CAD build for the part. Positions are in the model's coordinates, mm. A direction names the side the tool comes from. Give positions to 0.01 mm unless a question says otherwise; leave off trailing zeros. Order: outer loops, then holes, each group sorted by start corner. A loop starts at its lowest first (then second) coordinate and runs counter-clockwise, first axis right, second up.
Item 1: Two-plate mould, pull along X, no slides. Class faces 1 (the flat face through (-1.386, 0.74, 5.223)), 2 (the flat face through (0.1, 0, 2.5)), 3 (the flat face through (-5.328, 0.74, 0.835)): released by +X, released by -X, zero draft, split by the parting line, or undercut.
Item 2: Band-saw the part on A-A on x = 0. Give the cut face in (y, z).
Item 3: Which spindle directions (+Z, -Z, +X, -X, +Y, -Y) get a long thin tool onto all of the face, cutting with end or side? Do faces 4 (the flat face through (2.44, 0.74, 4.81)), 5 (the flat face through (-1.387, 0.74, -5.211)), 6 (the flat face through (-5.34, 0.74, -0.83)), 7 (the flat face through (1.387, 0.74, 5.211)). Say none if no direction does.
Item 4: Band-saw the part on B-B on z = -1.5. Give the cut face in (x, y), plus the area to 3 significant figures.
Item 5: Flat gauge pins, fed straight in: P1, Ø3.5, axis at x = 0, z = 0, coming from the -Y side; P2, Ø2, axis at x = -4, z = 2.5, coming from the -Y side. Where does each tip first touch, or does it go through?
Item 6: Wall check: L1, parallel to X at y = 0.5, z = 0; L2, parallel to Z at x = 0.5, y = 1.1; L3, parallel to Z at x = -1, y = 0.15. Give the ranges that are in metal, low to high.
```python
from build123d import *

# Parameters (mm, degrees)
BOSS_EXTRUDE1_DEPTH = 1.5
SKETCH2_R           = 2
CUT_EXTRUDE1_DEPTH  = 9.326084366


with BuildPart() as part:
    # Sketch1 → Boss-Extrude1 (new body)
    with BuildSketch(Plane(origin=(0, 0, 0), x_dir=(1, 0, 0), z_dir=(0, 1, 0))):
        with BuildLine():
            Line((-0.133547548, 5.8), (0.133547548, 5.8))
            Line((0.133547548, 5.8), (0.408993174, 4.983244383))
            ThreePointArc((0.408993174, 4.983244383), (0.522642316, 4.972609477), (0.636019074, 4.959383))
            Line((0.636019074, 4.959383), (1.075258593, 5.701022181))
            Line((1.075258593, 5.701022181), (1.33651702, 5.645489988))
            Line((1.33651702, 5.645489988), (1.436130457, 4.789314075))
            ThreePointArc((1.436130457, 4.789314075), (1.545084972, 4.755282581), (1.653234236, 4.718772781))
            Line((1.653234236, 4.718772781), (2.237070774, 5.352882336))
            Line((2.237070774, 5.352882336), (2.481074286, 5.244244973))
            Line((2.481074286, 5.244244973), (2.400501948, 4.38606776))
            ThreePointArc((2.400501948, 4.38606776), (2.5, 4.330127019), (2.598195129, 4.271929549))
            Line((2.598195129, 4.271929549), (3.301112228, 4.770795846))
            Line((3.301112228, 4.770795846), (3.517196699, 4.613801288))
            Line((3.517196699, 4.613801288), (3.259959985, 3.791129237))
            ThreePointArc((3.259959985, 3.791129237), (3.345653032, 3.715724127), (3.429602427, 3.638382497))
            Line((3.429602427, 3.638382497), (4.220879236, 3.980202686))
            Line((4.220879236, 3.980202686), (4.399600739, 3.781712348))
            Line((4.399600739, 3.781712348), (3.976942128, 3.030500175))
            ThreePointArc((3.976942128, 3.030500175), (4.045084972, 2.938926261), (4.111119642, 2.84582067))
            Line((4.111119642, 2.84582067), (4.956173568, 3.015655569))
            Line((4.956173568, 3.015655569), (5.089721116, 2.784344431))
            Line((5.089721116, 2.784344431), (4.520112816, 2.137423713))
            ThreePointArc((4.520112816, 2.137423713), (4.567727288, 2.033683215), (4.612961202, 1.928882825))
            Line((4.612961202, 1.928882825), (5.474859333, 1.919309833))
            Line((5.474859333, 1.919309833), (5.557396256, 1.665287302))
            Line((5.557396256, 1.665287302), (4.865732884, 1.150931578))
            ThreePointArc((4.865732884, 1.150931578), (4.890738004, 1.039558454), (4.913194221, 0.927643544))
            Line((4.913194221, 0.927643544), (5.754267473, 0.739081047))
            Line((5.754267473, 0.739081047), (5.782186513, 0.473449127))
            Line((5.782186513, 0.473449127), (4.998697077, 0.114138211))
            ThreePointArc((4.998697077, 0.114138211), (5, 0), (4.998697077, -0.114138211))
            Line((4.998697077, -0.114138211), (5.782186513, -0.473449127))
            Line((5.782186513, -0.473449127), (5.754267473, -0.739081047))
            Line((5.754267473, -0.739081047), (4.913194221, -0.927643544))
            ThreePointArc((4.913194221, -0.927643544), (4.890738004, -1.039558454), (4.865732884, -1.150931578))
            Line((4.865732884, -1.150931578), (5.557396256, -1.665287302))
            Line((5.557396256, -1.665287302), (5.474859333, -1.919309833))
            Line((5.474859333, -1.919309833), (4.612961202, -1.928882825))
            ThreePointArc((4.612961202, -1.928882825), (4.567727288, -2.033683215), (4.520112816, -2.137423713))
            Line((4.520112816, -2.137423713), (5.089721116, -2.784344431))
            Line((5.089721116, -2.784344431), (4.956173568, -3.015655569))
            Line((4.956173568, -3.015655569), (4.111119642, -2.84582067))
            ThreePointArc((4.111119642, -2.84582067), (4.045084972, -2.938926261), (3.976942128, -3.030500175))
            Line((3.976942128, -3.030500175), (4.399600739, -3.781712348))
            Line((4.399600739, -3.781712348), (4.220879236, -3.980202686))
            Line((4.220879236, -3.980202686), (3.429602427, -3.638382497))
            ThreePointArc((3.429602427, -3.638382497), (3.345653032, -3.715724127), (3.259959985, -3.791129237))
            Line((3.259959985, -3.791129237), (3.517196699, -4.613801288))
            Line((3.517196699, -4.613801288), (3.301112228, -4.770795846))
            Line((3.301112228, -4.770795846), (2.598195129, -4.271929549))
            ThreePointArc((2.598195129, -4.271929549), (2.5, -4.330127019), (2.400501948, -4.38606776))
            Line((2.400501948, -4.38606776), (2.481074286, -5.244244973))
            Line((2.481074286, -5.244244973), (2.237070774, -5.352882336))
            Line((2.237070774, -5.352882336), (1.653234236, -4.718772781))
            ThreePointArc((1.653234236, -4.718772781), (1.545084972, -4.755282581), (1.436130457, -4.789314075))
            Line((1.436130457, -4.789314075), (1.33651702, -5.645489988))
            Line((1.33651702, -5.645489988), (1.075258593, -5.701022181))
            Line((1.075258593, -5.701022181), (0.636019074, -4.959383))
            ThreePointArc((0.636019074, -4.959383), (0.522642316, -4.972609477), (0.408993174, -4.983244383))
            Line((0.408993174, -4.983244383), (0.133547548, -5.8))
            Line((0.133547548, -5.8), (-0.133547548, -5.8))
            Line((-0.133547548, -5.8), (-0.408993174, -4.983244383))
            ThreePointArc((-0.408993174, -4.983244383), (-0.522642316, -4.972609477), (-0.636019074, -4.959383))
            Line((-0.636019074, -4.959383), (-1.075258593, -5.701022181))
            Line((-1.075258593, -5.701022181), (-1.33651702, -5.645489988))
            Line((-1.33651702, -5.645489988), (-1.436130457, -4.789314075))
            ThreePointArc((-1.436130457, -4.789314075), (-1.545084972, -4.755282581), (-1.653234236, -4.718772781))
            Line((-1.653234236, -4.718772781), (-2.237070774, -5.352882336))
            Line((-2.237070774, -5.352882336), (-2.481074286, -5.244244973))
            Line((-2.481074286, -5.244244973), (-2.400501948, -4.38606776))
            ThreePointArc((-2.400501948, -4.38606776), (-2.5, -4.330127019), (-2.598195129, -4.271929549))
            Line((-2.598195129, -4.271929549), (-3.301112228, -4.770795846))
            Line((-3.301112228, -4.770795846), (-3.517196699, -4.613801288))
            Line((-3.517196699, -4.613801288), (-3.259959985, -3.791129237))
            ThreePointArc((-3.259959985, -3.791129237), (-3.345653032, -3.715724127), (-3.429602427, -3.638382497))
            Line((-3.429602427, -3.638382497), (-4.220879236, -3.980202686))
            Line((-4.220879236, -3.980202686), (-4.399600739, -3.781712348))
            Line((-4.399600739, -3.781712348), (-3.976942128, -3.030500175))
            ThreePointArc((-3.976942128, -3.030500175), (-4.045084972, -2.938926261), (-4.111119642, -2.84582067))
            Line((-4.111119642, -2.84582067), (-4.956173568, -3.015655569))
            Line((-4.956173568, -3.015655569), (-5.089721116, -2.784344431))
            Line((-5.089721116, -2.784344431), (-4.520112816, -2.137423713))
            ThreePointArc((-4.520112816, -2.137423713), (-4.567727288, -2.033683215), (-4.612961202, -1.928882825))
            Line((-4.612961202, -1.928882825), (-5.474859333, -1.919309833))
            Line((-5.474859333, -1.919309833), (-5.557396256, -1.665287302))
            Line((-5.557396256, -1.665287302), (-4.865732884, -1.150931578))
            ThreePointArc((-4.865732884, -1.150931578), (-4.890738004, -1.039558454), (-4.913194221, -0.927643544))
            Line((-4.913194221, -0.927643544), (-5.754267473, -0.739081047))
            Line((-5.754267473, -0.739081047), (-5.782186513, -0.473449127))
            Line((-5.782186513, -0.473449127), (-4.998697077, -0.114138211))
            ThreePointArc((-4.998697077, -0.114138211), (-5, 0), (-4.998697077, 0.114138211))
            Line((-4.998697077, 0.114138211), (-5.782186513, 0.473449127))
            Line((-5.782186513, 0.473449127), (-5.754267473, 0.739081047))
            Line((-5.754267473, 0.739081047), (-4.913194221, 0.927643544))
            ThreePointArc((-4.913194221, 0.927643544), (-4.890738004, 1.039558454), (-4.865732884, 1.150931578))
            Line((-4.865732884, 1.150931578), (-5.557396256, 1.665287302))
            Line((-5.557396256, 1.665287302), (-5.474859333, 1.919309833))
            Line((-5.474859333, 1.919309833), (-4.612961202, 1.928882825))
            ThreePointArc((-4.612961202, 1.928882825), (-4.567727288, 2.033683215), (-4.520112816, 2.137423713))
            Line((-4.520112816, 2.137423713), (-5.089721116, 2.784344431))
            Line((-5.089721116, 2.784344431), (-4.956173568, 3.015655569))
            Line((-4.956173568, 3.015655569), (-4.111119642, 2.84582067))
            ThreePointArc((-4.111119642, 2.84582067), (-4.045084972, 2.938926261), (-3.976942128, 3.030500175))
            Line((-3.976942128, 3.030500175), (-4.399600739, 3.781712348))
            Line((-4.399600739, 3.781712348), (-4.220879236, 3.980202686))
            Line((-4.220879236, 3.980202686), (-3.429602427, 3.638382497))
            ThreePointArc((-3.429602427, 3.638382497), (-3.345653032, 3.715724127), (-3.259959985, 3.791129237))
            Line((-3.259959985, 3.791129237), (-3.517196699, 4.613801288))
            Line((-3.517196699, 4.613801288), (-3.301112228, 4.770795846))
            Line((-3.301112228, 4.770795846), (-2.598195129, 4.271929549))
            ThreePointArc((-2.598195129, 4.271929549), (-2.5, 4.330127019), (-2.400501948, 4.38606776))
            Line((-2.400501948, 4.38606776), (-2.481074286, 5.244244973))
            Line((-2.481074286, 5.244244973), (-2.237070774, 5.352882336))
            Line((-2.237070774, 5.352882336), (-1.653234236, 4.718772781))
            ThreePointArc((-1.653234236, 4.718772781), (-1.545084972, 4.755282581), (-1.436130457, 4.789314075))
            Line((-1.436130457, 4.789314075), (-1.33651702, 5.645489988))
            Line((-1.33651702, 5.645489988), (-1.075258593, 5.701022181))
            Line((-1.075258593, 5.701022181), (-0.636019074, 4.959383))
            ThreePointArc((-0.636019074, 4.959383), (-0.522642316, 4.972609477), (-0.408993174, 4.983244383))
            Line((-0.408993174, 4.983244383), (-0.133547548, 5.8))
        make_face()
    extrude(amount=BOSS_EXTRUDE1_DEPTH)

    # Sketch2 → Cut-Extrude1 (cut, through all)
    with BuildSketch(Plane(origin=(0, 1.5, 0), x_dir=(1, 0, 0), z_dir=(0, 1, 0))):
        with Locations(Location((0, 0, 0), (0, 0, 270))):
            Circle(SKETCH2_R)
    extrude(amount=-CUT_EXTRUDE1_DEPTH, mode=Mode.SUBTRACT)


solid = part.part
```
The answers:
1. face 1: undercut
1. face 2: zero draft
1. face 3: released by -X
2. outline: (0, -5.8) - (1.5, -5.8) - (1.5, -2) - (0, -2) - close; (0, 2) - (1.5, 2) - (1.5, 5.8) - (0, 5.8) - close
3. face 4: +Y, -Y
3. face 5: -Z, +Y, -Y
3. face 6: -X, +Y, -Y
3. face 7: +Z, +Y, -Y
4. outline: (-5.34, 0) - (-1.32, 0) - (-1.32, 1.5) - (-5.34, 1.5) - close; (1.32, 0) - (5.34, 0) - (5.34, 1.5) - (1.32, 1.5) - close
4. area: 12.0 mm2
5. P1: passes through
5. P2: stops at y = 0
6. L1: x = -5 to -2, 2 to 5
6. L2: z = -4.97 to -1.94, 1.94 to 4.97
6. L3: z = -5.57 to -1.73, 1.73 to 5.57
